from build123d import *

# Parameters (mm, degrees)
CYLINDER001_R     = 1.5
CYLINDER001_DEPTH = 30
ARRAY_COUNT       = 8
CYLINDER_R        = 8
CYLINDER_DEPTH    = 15
FILLET_R          = 2


with BuildPart() as array:
    # Cylinder001 → Cylinder001 (new body)
    with BuildSketch(Plane(origin=(7.5, 0, 0), x_dir=(1, 0, 0), z_dir=(0, 0, 1))):
        Circle(CYLINDER001_R)
    extrude(amount=CYLINDER001_DEPTH)

    # Array: Array ×8 about axis
    array_axis = Axis((0, 0, 0), (0, 0, 1))


with BuildPart() as array_1:
    add(array.part)
    for i in range(1, ARRAY_COUNT):
        add(array.part.rotate(array_axis, i * 360 / ARRAY_COUNT))


with BuildPart() as array_2:
    # Array placement: moved
    add(array_1.part.moved(Location((0, 0, 2))))


with BuildPart() as cut:
    # Cylinder → Cylinder (new body)
    with BuildSketch(Plane.XY):
        Circle(CYLINDER_R)
    extrude(amount=CYLINDER_DEPTH)

    # Fillet
    fillet_edges = [cut.edges().sort_by_distance(p)[0] for p in [
        (-8, 0, 15),
    ]]
    fillet(fillet_edges, radius=FILLET_R)

    # Cut: cut Array
    add(array_2.part, mode=Mode.SUBTRACT)


solid = cut.part
Build history of the part. All positions in model axes, mm. A direction names the side the tool comes from. Round coordinates to 2 decimals unless told otherwise and drop trailing zeros. Write each loop counter-clockwise with the first axis right and the second up, starting at its lowest first coordinate (ties: lowest second). Pieces come first, ordered by that corner, then holes. Notation, with made-up numbers: (77.5, 4.25) - (125.5, 4.25) arc R32 cw to (125.5, 31.25) - close; hole circle Ø7 at (24.5, -8.75). An arc over 180 degrees is marked (long way). Use CSV: the item, a comma, the result in double quotes.
(1) Mould opens along Y. For faces 1 (the flat face through (0, 0, 15)), 2 (the cylindrical face through (7.39, -3.06, 6.41)), 3 (the cylindrical face through (0, 6, 8)), 4 (the flat face through (-5, -5, 2)) say: pulls with the +Y half, pulls with the -Y half, needs draft (parallel to the pull), parting line crosses it, or undercut.
Response:
face 1,"needs draft"
face 2,"parting line crosses it"
face 3,"undercut"
face 4,"undercut"
(2) Wall check: line 1 (X direction, y = -6.75, z = 10); line 2 (Y direction, x = -0.75, z = 6); line 3 (X direction, y = 5.5, z = 4). Give the ranges that are in metal, low to high.
Response:
line 1,"-4.29 to -1.3, 1.3 to 4.29"
line 2,"-6.2 to 6.2"
line 3,"-3.82 to 3.82"
(3) Pin check, flat tips, straight feed: P1, Ø0.8, axis at x = -5, y = 5, coming from the +Z side; P2, Ø8, axis at x = 0, z = 6.5, coming from the -Y side; P3, Ø1, axis at y = -2, z = 7, coming from the -X side. Stop position of each tip, or through.
Response:
P1,"z = 2"
P2,"y = -7.87"
P3,"x = -7.86"
(4) 3-axis set-ups, long thin cutter, end or side, ignore diameter. For faces 5 (the cylindrical face through (-6, 0, 8)), 6 (the flat face through (0, 0, 0)): which of +Z, -Z, +X, -X, +Y, -Y reach the whole face in a straight line?
Response:
face 5,"+Z"
face 6,"-Z, +X, -X, +Y, -Y"
(5) Band-saw the part on A-A (z = 10). Write the cut outline in (x, y).
Response:
outline,"(-7.87, -1.45) arc R8 ccw to (-6.59, -4.53) arc R1.5 cw (long way) to (-4.53, -6.59) arc R8 ccw to (-1.45, -7.87) arc R1.5 cw (long way) to (1.45, -7.87) arc R8 ccw to (4.53, -6.59) arc R1.5 cw (long way) to (6.59, -4.53) arc R8 ccw to (7.87, -1.45) arc R1.5 cw (long way) to (7.87, 1.45) arc R8 ccw to (6.59, 4.53) arc R1.5 cw (long way) to (4.53, 6.59) arc R8 ccw to (1.45, 7.87) arc R1.5 cw (long way) to (-1.45, 7.87) arc R8 ccw to (-4.53, 6.59) arc R1.5 cw (long way) to (-6.59, 4.53) arc R8 ccw to (-7.87, 1.45) arc R1.5 cw (long way) to start"
